Geometry check sheet. Reference: drawing and pictorial views, mm from the part's lowest x, y, z. Coordinates: 2 decimals unless noted, no trailing zeros. Order: outer loops, then holes, each group sorted by start corner. A loop starts at its lowest first (then second) coordinate and runs counter-clockwise, first axis right, second up. Notation, with made-up numbers: M -15.75,88.5 L -10.75,88.5 A7 cw -10.75,98.5 Z; hole C 81.5,-33 d9. An arc over 180 degrees is marked long. Return JSON: item names as keys, results as strings.
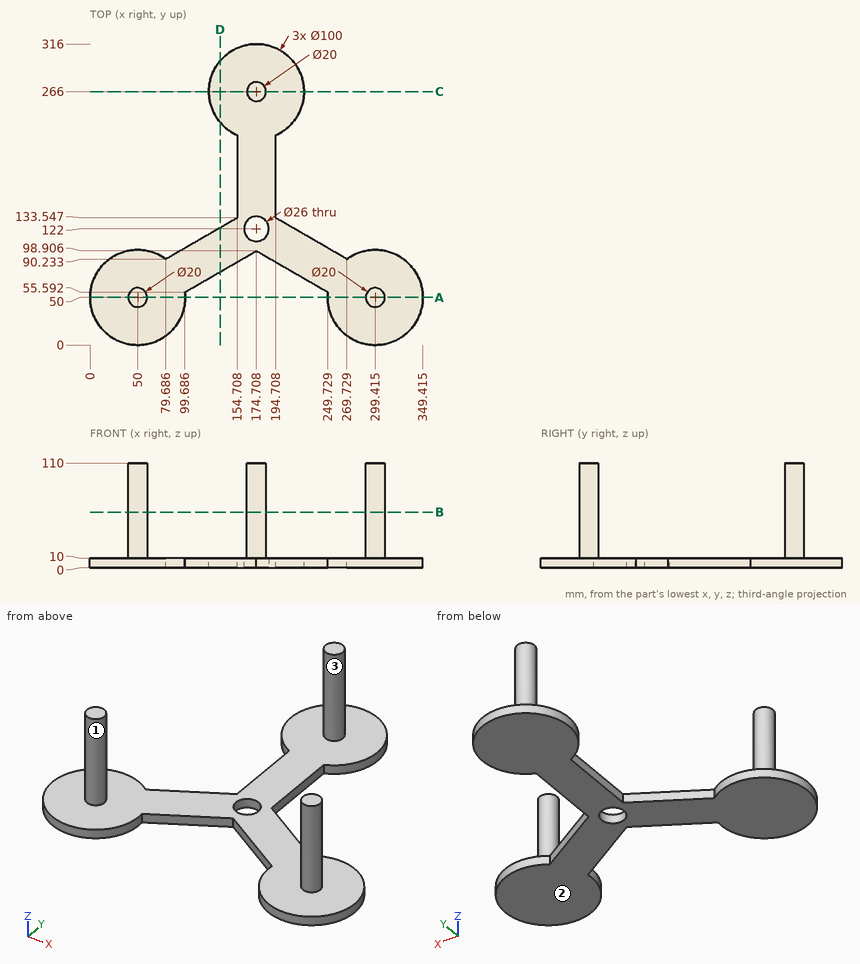
Q1. Cross-section at D-D, the plane x = 136.5. Record the boundary of the cut face in (y, z) (1 decimal).
Values:
{"outline": "M 76.8,0 L 123,0 L 123,10 L 76.8,10 Z; M 233.7,0 L 298.3,0 L 298.3,10 L 233.7,10 Z"}
Q2. Material ranges on line 1 along Z through (x, y) = (224.5, 84); line 2 along Y through (x, z) = (47, 43); line 3 along Y through (x, z) = (167, 103.5), recorded low to high.
Values:
{"line 1": "0 to 10", "line 2": "40.46 to 59.54", "line 3": "259.63 to 272.37"}
Q3. Draft check along X on the marked faces 1, 2 and 3. Enter one of: pulls with the +X half, pulls with the -X half, needs draft (parallel to the pull), parting line crosses it, or undercut.
Values:
{"face 1": "undercut", "face 2": "needs draft", "face 3": "parting line crosses it"}
Q4. Cross-section at B-B, the plane z = 58.5. Record the boundary of the cut face in (x, y) (1 decimal).
Values:
{"outline": "C 50,50 d20; C 174.7,266 d20; C 299.4,50 d20"}
Q5. Cross-section at C-C, the plane y = 266. Record the boundary of the cut face in (x, z), and give its area (3 significant figures).
Values:
{"outline": "M 124.71,0 L 224.71,0 L 224.71,10 L 184.71,10 L 184.71,110 L 164.71,110 L 164.71,10 L 124.71,10 Z", "area": "3,000 mm^2"}
Q6. Cross-section at A-A, the plane y = 50. Record the boundary of the cut face in (x, z) (1 decimal), and give its area (3 significant figures).
Values:
{"outline": "M 0,0 L 100,0 L 100,10 L 60,10 L 60,110 L 40,110 L 40,10 L 0,10 Z; M 249.4,0 L 349.4,0 L 349.4,10 L 309.4,10 L 309.4,110 L 289.4,110 L 289.4,10 L 249.4,10 Z", "area": "6,000 mm^2"}
Q7. Go/stop test with flat-tipped pins: pin 1 (8 mm diameter, centred on y = 157, z = 6, fed in from -X); pin 2 (10 mm diameter, centred on x = 38, y = 73.5, fed in from -Z); pin 3 (10 mm diameter, centred on x = 170, y = 232, fed in from +Z); pin 4 (8 mm diameter, centred on y = 192, z = 7, fed in from +X). Record where each tip stops, or that it passes through.
Values:
{"pin 1": "x = 154.71", "pin 2": "z = 0", "pin 3": "z = 10", "pin 4": "x = 194.71"}
